Design review of the part built by this model. Coordinates are the model's own, in mm. Coordinates: 2 decimals unless noted, no trailing zeros. Order: outer loops, then holes, each group sorted by start corner. A loop starts at its lowest first (then second) coordinate and runs counter-clockwise, first axis right, second up. Notation, with made-up numbers: M 66,36 L 107,36 A9 ccw 107,45 Z; hole C 29.5,31.25 d3. An arc over 180 degrees is marked long. Use CSV: the item, a comma, the result in double quotes.
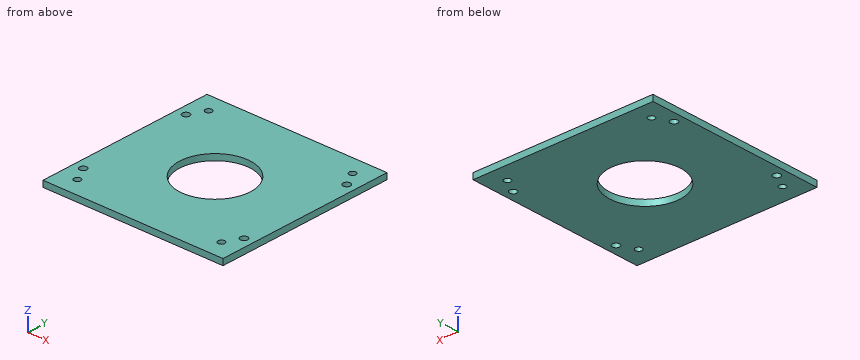
```python
from build123d import *

# Parameters (mm, degrees)
F2_W            = 150
F2_H            = 150
F2_R            = 29.5
F3_DEPTH        = 5
F5_D            = 5.5
F5_COPIES_COUNT = 4
F6_R            = 3
F7_DEPTH        = 5.001


# Not quite as in the source:
# - a pattern or mirror of a feature is missing from the dataset's text; its kind, count and spacing are read off the source's solid
# - a feature names something its author has since deleted; it is built from what else it names


with BuildPart() as f3:
    # F2 (on Top) → F3 (new body)
    with BuildSketch(Plane.XY):
        Rectangle(F2_W, F2_H)
        Circle(F2_R, mode=Mode.SUBTRACT)
    extrude(amount=-F3_DEPTH)

    # F5 (through all)
    with Locations(Plane.XY):
        with Locations((-60, -60)):
            f5 = Hole(F5_D / 2)

    # F5_copies: F5 ×4 about axis
    f5_copies_axis = Axis((0, 0, 0), (0, 0, 1))
    for i in range(1, F5_COPIES_COUNT):
        add(f5.rotate(f5_copies_axis, i * 360 / F5_COPIES_COUNT), mode=Mode.SUBTRACT)

    # F6 (on Top) → F7 (cut, through all)
    with BuildSketch(Plane.XY):
        with Locations((-67, -47)):
            Circle(F6_R)
    f7 = extrude(amount=-F7_DEPTH, mode=Mode.SUBTRACT)

    # F7_copies: F7 across plane
    add(f7.mirror(Plane(origin=(0, 0, 0), x_dir=(0, 0, 1), z_dir=(1, 0, 0))), mode=Mode.SUBTRACT)

    # F7_copies1: F7 across plane
    add(f7.mirror(Plane.ZX), mode=Mode.SUBTRACT)

    # F7_copies2: F7 across plane
    add(f7.mirror(Plane(origin=(0, 0, 0), x_dir=(-0.5742821086, 0.818657474, 0), z_dir=(0.818657474, 0.5742821086, 0))), mode=Mode.SUBTRACT)


solid = f3.part
```
(1) Wall thickness on probe 1 along X at (y, z) = (47, -2.7); probe 2 along Y at (x, z) = (67, -2.25); probe 3 along Y at (x, z) = (60, -2.25): over which ranges is each line inside the solid? List them lowest first.
The answers:
probe 1,"x = -75 to -70, -64 to 64, 70 to 75"
probe 2,"y = -75 to -50, -44 to 44, 50 to 75"
probe 3,"y = -75 to -62.75, -57.25 to 57.25, 62.75 to 75"
(2) Add section D-D on y = -20.5. State the section outline as (x, z) points.
The answers:
outline,"M -75,-5 L -21.21,-5 L -21.21,0 L -75,0 Z; M 21.21,-5 L 75,-5 L 75,0 L 21.21,0 Z"
(3) Add section C-C on x = -11.5. State the section outline as (y, z) points.
The answers:
outline,"M -75,-5 L -27.17,-5 L -27.17,0 L -75,0 Z; M 27.17,-5 L 75,-5 L 75,0 L 27.17,0 Z"
(4) Add section A-A on x = 60. State the section outline as (y, z) points.
The answers:
outline,"M -75,-5 L -62.75,-5 L -62.75,0 L -75,0 Z; M -57.25,-5 L 57.25,-5 L 57.25,0 L -57.25,0 Z; M 62.75,-5 L 75,-5 L 75,0 L 62.75,0 Z"
